Autodesk Inventor part; units mm, degrees
ref_plane "Work Plane1" through (0, 0, 0) normal (0, 0, 1) x (1, 0, 0)
ref_plane "YZ Plane" through (0, 0, 0) normal (1, 0, 0) x (0, 1, 0)
ref_plane "XZ Plane" through (0, 0, 0) normal (0, 1, 0) x (-1, 0, 0)
ref_plane "Work Plane1" through (0, 0, 0) normal (0, 0, 1) x (1, 0, 0)
sketch "Sketch1" plane through (0, 0, 0) normal (0, 0, 1) x (1, 0, 0)
  circle A0 centre (-17.75, 4.5) radius 1.5
  arc A1 (-25.75, 8) -> (-27.75, 6) centre (-25.75, 6) ccw
  line L0 (-27.75, 3) -> (-27.75, 6)
  line L1 (-30.85, 1) -> (-29.75, 1)
  arc A2 (-30.85, 1) -> (-32.85, -1) centre (-30.85, -1) ccw
  line L2 (-32.85, -13) -> (-32.85, -1)
  arc A3 (-32.85, -13) -> (-30.85, -15) centre (-30.85, -13) ccw
  line L3 (5.15, -15) -> (-30.85, -15)
  arc A4 (5.15, -15) -> (7.15, -13) centre (5.15, -13) ccw
  line L4 (7.15, -1) -> (7.15, -13)
  arc A5 (7.15, -1) -> (5.15, 1) centre (5.15, -1) ccw
  line L5 (-30.85, 1) -> (5.15, 1)
  line L6 (-7.75, 3) -> (-7.75, 6)
  arc A6 (-7.75, 6) -> (-9.75, 8) centre (-9.75, 6) ccw
  line L7 (-25.75, 8) -> (-9.75, 8)
  circle A7 centre (-8.75, -7) radius 1.5
  circle A8 centre (-26.75, -7) radius 1.5
  line L8 (-30.85, -12) -> (-5.5342, -12)
  line L9 (-30.85, -2) -> (-30.85, -12)
  line L10 (-5.5342, -2) -> (-5.5342, -12)
  line L11 (-5.5342, -2) -> (-30.85, -2)
  line L12 (-11.5342, -2) -> (-11.5342, -12)
  line L13 (-23.85, -2) -> (-23.85, -12)
  point P0 (0, 0)
  dimension "d2" = 6
  dimension "d3" = 12.6842
  dimension "d4" = 2
  dimension "d5" = 7
extrude "Extrusion4" add sketch "Sketch1" along normal blind 5.2 contours L1 L5 A5 L4 A4 L3 A3 L2 A2
sketch "Sketch5" plane through (0, 0, 5.2) normal (0, 0, 1) x (1, 0, 0)
  line L0 (-30.85, -3) -> (-23.85, -3)
  line L1 (-5.5342, -3) -> (-5.5342, -11)
  line L2 (-5.5342, -11) -> (-11.5342, -11)
  line L3 (-30.85, -11) -> (-30.85, -3)
  arc A0 (-30.85, 1) -> (-32.85, -1) centre (-30.85, -1) ccw
  line L4 (-32.85, -1) -> (-32.85, -13)
  arc A1 (-32.85, -13) -> (-30.85, -15) centre (-30.85, -13) ccw
  line L5 (-30.85, -15) -> (5.15, -15)
  arc A2 (5.15, -15) -> (7.15, -13) centre (5.15, -13) ccw
  line L6 (7.15, -13) -> (7.15, -1)
  arc A3 (7.15, -1) -> (5.15, 1) centre (5.15, -1) ccw
  line L7 (5.15, 1) -> (-30.85, 1)
  line L8 (-11.5342, -15) -> (-11.5342, 1)
  line L9 (-23.85, -15) -> (-23.85, 1)
  circle A4 centre (-8.75, -7) radius 1.5
  circle A5 centre (-26.75, -7) radius 1.5
  line L10 (-11.5342, -3) -> (-5.5342, -3)
  line L11 (-23.85, -3) -> (-11.5342, -3)
  line L12 (-11.5342, -11) -> (-23.85, -11)
  line L13 (-23.85, -11) -> (-30.85, -11)
  point P0 (0, 0)
  point P1 (-11.5342, -14)
  point P2 (-11.5342, 2)
  point P3 (-23.85, -14)
  point P4 (-23.85, 2)
  dimension "d16" = 6
  dimension "d17" = 7
  dimension "d22" = 4
  dimension "d23" = 4
extrude "Extrusion5" add sketch "Sketch5" along normal blind 3 contours L3 L13 L9 L5 A1 L4 A0 L7 L0 | L0 L9 L13 L3 | L9 L7 L8 L11 | L12 L8 L5 L9 | L10 L1 L2 L8 | L8 L7 A3 L6 A2 L5 L2 L1 L10
sketch "Sketch6" plane through (0, 0, 8.2) normal (0, 0, 1) x (1, 0, 0)
  line L0 (-16.35, -15) -> (-16.35, 1)
  line L1 (-19.15, -15) -> (-19.15, 1)
  line L2 (5.15, 1) -> (-30.85, 1)
  line L3 (-30.85, -15) -> (5.15, -15)
  point P0 (0, 0)
extrude "Extrusion6" cut sketch "Sketch6" against normal blind 4
sketch "Sketch7" plane through (0, 0, 0) normal (0, 0, -1) x (-1, 0, 0)
  line L0 (5.5342, -2) -> (30.85, -2)
  line L1 (30.85, -2) -> (30.85, -12)
  line L2 (30.85, -12) -> (5.5342, -12)
  line L3 (5.5342, -12) -> (5.5342, -2)
  line L4 (4.0342, -12.7) -> (31.55, -12.7)
  line L5 (31.55, -12.7) -> (31.55, -1.3)
  line L6 (31.55, -1.3) -> (4.0342, -1.3)
  line L7 (4.0342, -1.3) -> (4.0342, -12.7)
  line L8 (4.0342, -12.7) -> (-5.2525, -12.7)
  line L9 (-5.2525, -12.7) -> (-5.2525, -1.7)
  line L10 (-5.2525, -1.7) -> (4.0342, -1.7)
  line L11 (4.0342, -1.7) -> (4.0342, -12.7)
  point P0 (0, 0)
  dimension "d24" = 0.7
  dimension "d31" = 1.5
extrude "Extrusion7" cut sketch "Sketch7" against normal blind 5.2
sketch "Sketch8" plane through (0, 0, 8.2) normal (0, 0, 1) x (1, 0, 0)
  circle A0 centre (-3.75, -7.199) radius 1
  circle A1 centre (-8.75, -7) radius 1.5
  point P0 (0, 0)
  dimension "d27" = 2
  dimension "d28" = 5
extrude "Extrusion8" cut sketch "Sketch8" against normal through all contours A0
properties part number "optical endstop top"
The model under review builds one solid part; all positions refer to its coordinate system, in mm. A direction names the side the tool comes from. Round coordinates to 2 decimals unless told otherwise and drop trailing zeros. Loops run counter-clockwise (first coordinate to the right, second up) from the corner with the lowest first, then second, coordinate; pieces in that order, holes last.
Item 1: For line 1 (Y direction, x = -2.5, z = 2); line 2 (Y direction, x = -19.5, z = 6); line 3 (X direction, y = -6.5, z = 5), list the stretches that pass through material, from the lowest coordinate up.
Determined:
line 1: y = -15 to -12.7, -1.7 to 1
line 2: y = -15 to -11, -3 to 1
line 3: x = -32.85 to -31.55, 5.25 to 7.15
Item 2: Clearance check with flat-ended pins moving along their axes: pin 1 Ø4.5 at (y, z) = (-14, 7) entering from -X; pin 2 Ø3.5 at (x, y) = (-24, -9) entering from -Z. State where each tip first meets the part, or that it passes through.
Determined:
pin 1: stops at x = -32.85
pin 2: stops at z = 5.2
Item 3: Take a section at A-A (x = -8.75). Write out the cut boundary in (y, z), then the cut area to 3 significant figures.
Determined:
outline: (-15, 0) - (-12.7, 0) - (-12.7, 5.2) - (-8.5, 5.2) - (-8.5, 8.2) - (-15, 8.2) - close; (-5.5, 5.2) - (-1.3, 5.2) - (-1.3, 0) - (1, 0) - (1, 8.2) - (-5.5, 8.2) - close
area: 62.9 mm2
Item 4: Mouldability with a two-part tool opening along Y and no side actions: class faces 4 (the face through (-19.15, -13, 6)), 5 (the face through (1, -1.7, 3)), 6 (the face through (-13, -15, 4)), 7 (the face through (-32.28, 0.4, 4.04)) as released by +Y, released by -Y, zero draft, split by the parting line, or undercut.
Determined:
face 4: zero draft
face 5: undercut
face 6: released by -Y
face 7: released by +Y
Item 5: Take a section at C-C (z = 7). Write out the cut boundary in (x, y).
Determined:
outline: (-32.85, -13) arc R2 ccw to (-30.85, -15) - (-19.15, -15) - (-19.15, -11) - (-23.85, -11) - (-23.85, -3) - (-19.15, -3) - (-19.15, 1) - (-30.85, 1) arc R2 ccw to (-32.85, -1) - close; (-16.35, -15) - (5.15, -15) arc R2 ccw to (7.15, -13) - (7.15, -1) arc R2 ccw to (5.15, 1) - (-16.35, 1) - (-16.35, -3) - (-11.53, -3) - (-11.53, -11) - (-16.35, -11) - close; hole circle Ø3 at (-26.75, -7); hole circle Ø3 at (-8.75, -7); hole circle Ø2 at (-3.75, -7.2)
Item 6: For faces 1 (the face through (-31.55, -7, 3)), 2 (the face through (-21, -11, 7)), 3 (the face through (-16.35, -1, 6)), list the 3-axis set-ups (+Z, -Z, +X, -X, +Y, -Y) from which the entire face can be reached by the end or side of a thin tool; tool diameter is ignored.
Determined:
face 1: -Z
face 2: +Z, -Z
face 3: +Z, +Y, -Y
Item 7: Take a section at B-B (y = -10.5). Write out the cut boundary in (x, z).
Determined:
outline: (-32.85, 0) - (-31.55, 0) - (-31.55, 5.2) - (-23.85, 5.2) - (-23.85, 8.2) - (-32.85, 8.2) - close; (-11.53, 5.2) - (5.25, 5.2) - (5.25, 0) - (7.15, 0) - (7.15, 8.2) - (-11.53, 8.2) - close
Item 8: Take a section at D-D (z = 1.75). Write out the cut boundary in (x, y).
Determined:
outline: (-32.85, -13) arc R2 ccw to (-30.85, -15) - (5.15, -15) arc R2 ccw to (7.15, -13) - (7.15, -1) arc R2 ccw to (5.15, 1) - (-30.85, 1) arc R2 ccw to (-32.85, -1) - close; hole (-31.55, -12.7) - (5.25, -12.7) - (5.25, -1.7) - (-4.03, -1.7) - (-4.03, -1.3) - (-31.55, -1.3) - close
